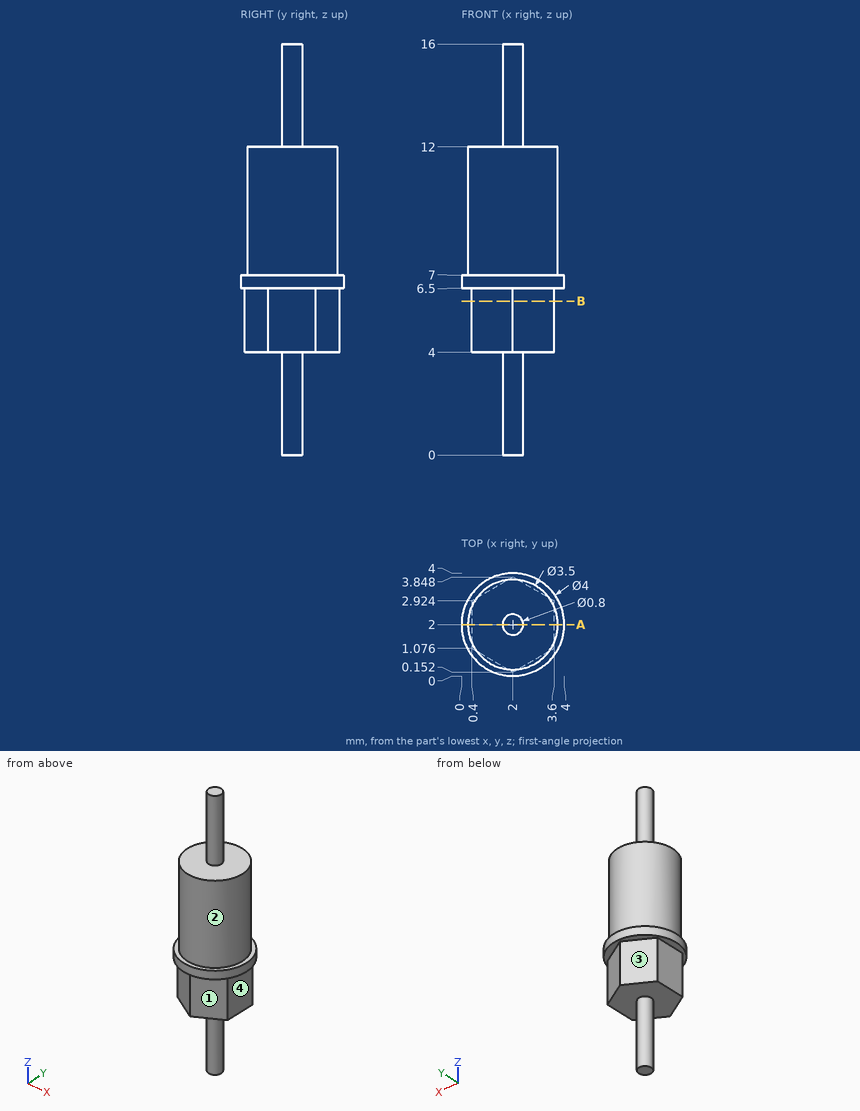
For this review, use the dimensioned drawing (mm, ordinates from the lowest corner) and the shaded views. A direction names the side the tool comes from. Coordinates: 2 decimals unless noted, no trailing zeros. Order: outer loops, then holes, each group sorted by start corner. A loop starts at its lowest first (then second) coordinate and runs counter-clockwise, first axis right, second up. Notation, with made-up numbers: M 45.25,49.25 L 51.25,49.25 A15 ccw 51.25,70.25 Z; hole C -10.75,39 d11. An arc over 180 degrees is marked long. Answer as a JSON object with one key per item and string values. Group by question number.
1) Add section A-A, the plane y = 2. Write out the cut boundary in (x, z), then the cut area to 3 significant figures.
2) Add section B-B, the plane z = 6. Write out the cut boundary in (x, y).
3) Wall thickness on L1, parallel to Z at x = 2.65, y = 2.95; L2, parallel to X at y = 2.85, z = 6; L3, parallel to Y at x = 3.1, z = 5.75: over which ranges is each line inside the solid? List them lowest first.
4) Tool access review of the marked faces 1, 2, 3 and 4: name each direction out of +Z, -Z, +X, -X, +Y, -Y from which nothing blocks a thin tool from reaching the whole face with its end or side.
5) For pin 1 (1 mm diameter, centred on y = 3.5, z = 2.5, fed in from +X); pin 2 (1.5 mm diameter, centred on y = 2, z = 5, fed in from +X); pin 3 (0.9 mm diameter, centred on y = 2, z = 5, fed in from -X); pin 4 (2 mm diameter, centred on y = 1.5, z = 13.5, fed in from +X), all flat-tipped, find the tip position at first contact; note any pin that passes through.
Computed values:
{
 "1": {"outline": "M 0,6.5 L 0.4,6.5 L 0.4,4 L 1.6,4 L 1.6,0 L 2.4,0 L 2.4,4 L 3.6,4 L 3.6,6.5 L 4,6.5 L 4,7 L 3.75,7 L 3.75,12 L 2.4,12 L 2.4,16 L 1.6,16 L 1.6,12 L 0.25,12 L 0.25,7 L 0,7 Z", "area": "33.9 mm^2"},
 "2": {"outline": "M 0.4,1.08 L 2,0.15 L 3.6,1.08 L 3.6,2.92 L 2,3.85 L 0.4,2.92 Z"},
 "3": {"L1": "z = 4 to 12", "L2": "x = 0.4 to 3.6", "L3": "y = 0.79 to 3.21"},
 "4": {"face 1": "-Z, +X, -Y", "face 2": "+Z", "face 3": "-Z, -X, +Y", "face 4": "-Z, +X, +Y, -Y"},
 "5": {"pin 1": "passes through", "pin 2": "stops at x = 3.6", "pin 3": "stops at x = 0.4", "pin 4": "stops at x = 2.4"}
}
